Build history of the part. All positions in model axes, mm. Face numbers are marked on the shaded views. A direction names the side the tool comes from. Round coordinates to 2 decimals unless told otherwise and drop trailing zeros. Loops run counter-clockwise (first coordinate to the right, second up) from the corner with the lowest first, then second, coordinate; pieces in that order, holes last. Notation, with made-up numbers: (-36, 33.5) - (-30, 33.5) arc R3 ccw to (-30, 37.5) - close; hole circle Ø9 at (46, 14.5). An arc over 180 degrees is marked (long way). Put each result on its own line as item: value. Start each with the question number.
from build123d import *

# Parameters (mm, degrees)
SKETCH1_R               = 15
BOSS_EXTRUDE1_DEPTH     = 12
SKETCH13_R              = 7
BOSS_EXTRUDE3_DEPTH     = 13
CUT_EXTRUDE2_DEPTH      = 25.372115214
CUT_EXTRUDE2_DEPTH_BACK = 25.372115214
SKETCH2_R               = 5
CIRPATTERN1_COUNT       = 3


with BuildPart() as part:
    # Sketch1 → Boss-Extrude1 (new body)
    with BuildSketch(Plane(origin=(0, 0, 0), x_dir=(1, 0, 0), z_dir=(0, 1, 0))):
        with Locations(Location((0, 0, 0), (0, 0, 270))):
            Circle(SKETCH1_R)
    extrude(amount=BOSS_EXTRUDE1_DEPTH)

    # Sketch13 → Boss-Extrude3 (add)
    with BuildSketch(Plane(origin=(0, 0, 0), x_dir=(1, 0, 0), z_dir=(0, 1, 0))):
        with Locations(Location((0, 0, 0), (0, 0, 90))):
            Circle(SKETCH13_R)
    extrude(amount=BOSS_EXTRUDE3_DEPTH)

    # Sketch2 → Cut-Extrude2 (cut, two sides: drawn at the far end of the back side and taken through both)
    with BuildSketch(Plane(origin=(0, 12, 0), x_dir=(1, 0, 0), z_dir=(0, 1, 0)).offset(-CUT_EXTRUDE2_DEPTH_BACK)):
        with Locations(Location((0, 0, 0), (0, 0, 270))):
            Circle(SKETCH2_R)
    extrude(amount=CUT_EXTRUDE2_DEPTH + CUT_EXTRUDE2_DEPTH_BACK, mode=Mode.SUBTRACT)

    # Sketch16 → Ø4.0mm Dowel Hole1 (revolve, cut)
    with BuildSketch(Plane(origin=(0, 6, 15), x_dir=(0, -1, 0), z_dir=(1, 0, 0))):
        Polygon((0, 0), (0, 16.050506083), (1.75, 14.999), (1.75, 0), align=None)
    f_4_0mm_dowel_hole1 = revolve(axis=Axis((0, 6, 21.35), (0, 0, -1)), mode=Mode.SUBTRACT)

    # CirPattern1: Ø4.0mm Dowel Hole1 ×3 about axis
    cirpattern1_axis = Axis((0, 0, 0), (0, 1, 0))
    for i in range(1, CIRPATTERN1_COUNT):
        add(f_4_0mm_dowel_hole1.rotate(cirpattern1_axis, i * 360 / CIRPATTERN1_COUNT), mode=Mode.SUBTRACT)


solid = part.part
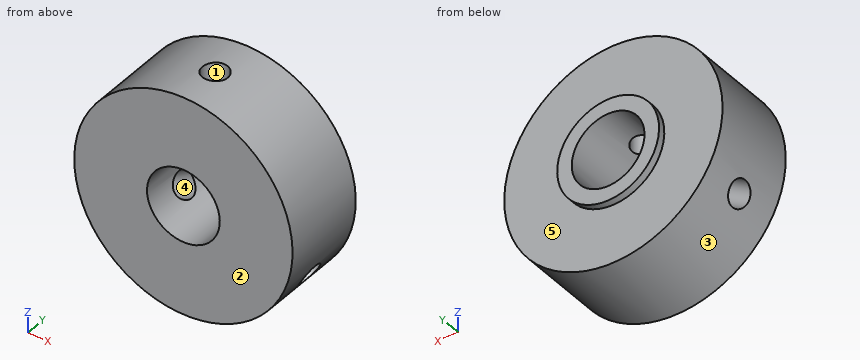
1) Slice it at D-D, the plane y = 1.75. Write the cut outline in (x, z).
2) Pull direction X, two halves, no side cores. Call the marked faces 1, 2 and 3: pulls with the +X half, pulls with the -X half, needs draft (parallel to the pull), parting line crosses it, or undercut.
3) Slice it at A-A, the plane z = 0. Write the cut outline in (x, y).
4) Slice it at B-B, the plane x = 0. Write the cut outline in (y, z), and give its area (3 significant figures).
5) Drop flat-ended pins along their axis: pin 1 Ø1.5 at (x, y) = (11.5, 7.5) entering from +Z; pin 2 Ø1 at (x, z) = (10, -10.5) entering from +Y; pin 3 Ø5 at (y, z) = (2, -10.5) entering from -X. Give the stop position or say it passes through.
6) Drill centre lines: line 1 (X direction, y = 9.5, z = 0); line 2 (Y direction, x = 0, z = 9); line 3 (Y direction, x = -7, z = 11.5). Where is each one in solid material? Low to high. Write a range as [from, to].
7) Slice it at C-C, the plane y = 6. Write the cut outline in (x, z).
8) Which spindle directions (+Z, -Z, +X, -X, +Y, -Y) get a long thin tool onto all of the face, cutting with end or side? Do the marked faces 4 and 5. Say none if no direction does.
Taken from the geometry:
1. outline: circle Ø30 at (0, 0); hole circle Ø10 at (0, 0)
2. face 1: undercut
2. face 2: needs draft
2. face 3: parting line crosses it
3. outline: (-15, 0) - (-5, 0) - (-5, 13) - (-7, 13) - (-7, 12) - (-15, 12) - close; (5, 0) - (15, 0) - (15, 12) - (7, 12) - (7, 13) - (5, 13) - close
4. outline: (0, -15) - (12, -15) - (12, -7) - (13, -7) - (13, -5) - (0, -5) - close; (0, 5) - (4.25, 5) - (4.25, 15) - (0, 15) - close; (7.75, 5) - (13, 5) - (13, 7) - (12, 7) - (12, 15) - (7.75, 15) - close
4. area: 209 mm2
5. pin 1: stops at z = 10.46
5. pin 2: stops at y = 12
5. pin 3: stops at x = -12.69
6. line 1: x = [-15, -5], [5, 15]
6. line 2: y = [0, 4.25], [7.75, 12]
6. line 3: y = [0, 12]
7. outline: (-13.78, -5.93) - (-4.93, -0.83) arc R5 cw to (-1.75, 4.68) - (-1.75, 14.9) arc R15 ccw to start; (-12.03, -8.96) arc R15 ccw to (12.03, -8.96) - (3.18, -3.86) arc R5 cw to (-3.18, -3.86) - close; (1.75, 4.68) arc R5 cw to (4.93, -0.83) - (13.78, -5.93) arc R15 ccw to (1.75, 14.9) - close
8. face 4: none
8. face 5: +Y
